Input: part model. Units: mm. Frame: model coordinates. A direction names the side the tool comes from. Coordinates: 2 decimals unless noted, no trailing zeros. Write each loop counter-clockwise with the first axis right and the second up, starting at its lowest first coordinate (ties: lowest second). Pieces come first, ordered by that corner, then holes. Notation, with made-up numbers: M -6,-6 L 32,-6 A15 cw 32,22 Z; hole C 80,28 d8. An arc over 180 degrees is marked long. Write each question's results on one line, items separated by ' | '. Start each with the question number.
1. Section query C-C, the plane x = -120. Output: boundary loops of the cut face in (y, z) (3 decimals).
2. Section query D-D, the plane z = -120. Output: boundary loops of the cut face in (x, y) (3 decimals).
3. First-contact query: pin 1 (6.5 mm diameter, centred on x = 103.92, z = 60, fed in from +Y); pin 2 (3 mm diameter, centred on x = 34, z = -78, fed in from -Y); pin 3 (1.5 mm diameter, centred on y = -21, z = -11.5, fed in from +X). Flat tips, straight axial feed; report the tip coordinate or a pass-through.
4. Ray query, probe 1 along Y at (x, z) = (-45.5, 20); probe 2 along X at (y, z) = (-3, -38); probe 3 along X at (y, z) = (-105.5, -60). Return the intervals inside material, ascending.
5. Pull-direction query (X, two-part tool) for faces 6 (the cylindrical face through (-103.207, -104.918, 65.453)), 7 (the flat face through (38.6, -14.265, -38.699)), 8 (the flat face through (-38.505, -85.33, -38.406)), 9 (the cylindrical face through (-44.74, 4.93, 101.49)); classes: +X half, -X half, draft (parallel to the pull), parting line (faces both ways), or undercut.
6. Set-up query: faces 1 (the flat face through (33.89, -91.01, -40.96)), 2 (the flat face through (38.406, -85.33, -38.505)), 3 (the flat face through (-29, 10, 29)), 4 (the cylindrical face through (98.677, -104.918, -58.348)), 5 (the flat face through (-38.56, -10.79, -31.49)). Return all of +Z, -Z, +X, -X, +Y, -Y with unobstructed straight access to the full face (end or side cutting, diameter ignored); none if empty.
7. Section query A-A, the plane y = 6.5. Count the separate pieces of the cut face and the enclosed holes in it, and give its area (3 significant figures).
8. Section query B-B, the plane z = -74.5. Output: boundary loops of the cut face in (x, y).
```python
from build123d import *

# Parameters (mm, degrees)
SKETCH_1_R                        = 140
SKETCH_1_R_2                      = 30
EXTRUDE_1_DEPTH                   = 10
HOLE_WIZARD_20_0_20_1_AT_2_COUNT  = 2
HOLE_WIZARD_20_0_20_1_AT_2_PITCH  = 127.279220614
HOLE_WIZARD_20_0_20_1_AT_3_COUNT  = 2
HOLE_WIZARD_20_0_20_1_AT_3_PITCH  = 180
HOLE_WIZARD_20_0_20_1_AT_4_COUNT  = 2
HOLE_WIZARD_20_0_20_1_AT_4_PITCH  = 127.279220614
SKETCH_4_R                        = 40
SKETCH_4_R_2                      = 30
EXTRUDE_2_DEPTH                   = 40
EXTRUDE_START                     = -100
SKETCH_6_R                        = 45
SKETCH_6_R_2                      = 30
EXTRUDE_3_DEPTH                   = 100
RIB_6_REACH                       = 223.811
SKETCH_7_WALL_W                   = 483.06475071
SKETCH_7_WALL_H                   = 10
PATTERN_CIRCULAR_1_COUNT          = 4
SKETCH_8_R                        = 131
EXTRUDE_4_DEPTH                   = 10
HOLE_WIZARD_11_0_11_1_D           = 11
HOLE_WIZARD_11_0_11_1_DEPTH       = 10
HOLE_WIZARD_11_0_11_1_CSINK_D     = 11.05
HOLE_WIZARD_11_0_11_1_CSINK_ANGLE = 90
RIB_7_REACH                       = 228.495
SKETCH_11_WALL_W                  = 492.43335657
SKETCH_11_WALL_H                  = 10
PATTERN_CIRCULAR_2_COUNT          = 4


with BuildPart() as part:
    # 草图1 → 凸台-拉伸1 (new body)
    with BuildSketch(Plane(origin=(0, 0, 0), x_dir=(1, 0, 0), z_dir=(0, 1, 0))):
        with Locations(Location((0, 0, 0), (0, 0, 270))):
            Circle(SKETCH_1_R)
        with Locations(Location((0, 0, 0), (0, 0, 270))):
            Circle(SKETCH_1_R_2, mode=Mode.SUBTRACT)
        with BuildLine():
            ThreePointArc((105.655099262, 61), (86.267027305, 86.267027305), (61, 105.655099262))
            ThreePointArc((61, 105.655099262), (44.607695155, 101.262794416), (49, 84.870489571))
            ThreePointArc((49, 84.870489571), (69.296464556, 69.296464556), (84.870489571, 49))
            ThreePointArc((84.870489571, 49), (101.262794416, 44.607695155), (105.655099262, 61))
        make_face(mode=Mode.SUBTRACT)
        with BuildLine():
            ThreePointArc((61, -105.655099262), (86.267027305, -86.267027305), (105.655099262, -61))
            ThreePointArc((105.655099262, -61), (101.262794416, -44.607695155), (84.870489571, -49))
            ThreePointArc((84.870489571, -49), (69.296464556, -69.296464556), (49, -84.870489571))
            ThreePointArc((49, -84.870489571), (44.607695155, -101.262794416), (61, -105.655099262))
        make_face(mode=Mode.SUBTRACT)
        with BuildLine():
            ThreePointArc((-105.655099262, -61), (-86.267027305, -86.267027305), (-61, -105.655099262))
            ThreePointArc((-61, -105.655099262), (-44.607695155, -101.262794416), (-49, -84.870489571))
            ThreePointArc((-49, -84.870489571), (-69.296464556, -69.296464556), (-84.870489571, -49))
            ThreePointArc((-84.870489571, -49), (-101.262794416, -44.607695155), (-105.655099262, -61))
        make_face(mode=Mode.SUBTRACT)
        with BuildLine():
            ThreePointArc((-61, 105.655099262), (-86.267027305, 86.267027305), (-105.655099262, 61))
            ThreePointArc((-105.655099262, 61), (-101.262794416, 44.607695155), (-84.870489571, 49))
            ThreePointArc((-84.870489571, 49), (-69.296464556, 69.296464556), (-49, 84.870489571))
            ThreePointArc((-49, 84.870489571), (-44.607695155, 101.262794416), (-61, 105.655099262))
        make_face(mode=Mode.SUBTRACT)
    extrude(amount=EXTRUDE_1_DEPTH)

    # 草图3 → Ø20.0 (20) 直径孔1 (revolve, cut)
    with BuildSketch(Plane(origin=(0, 10, 90), x_dir=(0, 0, 1), z_dir=(1, 0, 0))):
        Polygon((0, 0), (0, 10), (10, 10), (10, 0.025), (10.025, 0), align=None)
    hole_wizard_20_0_20_1 = revolve(axis=Axis((0, 16.35, 90), (0, -1, 0)), mode=Mode.SUBTRACT)

    # Ø20.0 (20) 直径孔1 at 2: Ø20.0 (20) 直径孔1 ×2
    with Locations(*[Vector(0.7071067811865476, 0, -0.7071067811865476) * (i * HOLE_WIZARD_20_0_20_1_AT_2_PITCH) for i in range(1, HOLE_WIZARD_20_0_20_1_AT_2_COUNT)]):
        add(hole_wizard_20_0_20_1, mode=Mode.SUBTRACT)

    # Ø20.0 (20) 直径孔1 at 3: Ø20.0 (20) 直径孔1 ×2
    with Locations(*[(0, 0, -i * HOLE_WIZARD_20_0_20_1_AT_3_PITCH) for i in range(1, HOLE_WIZARD_20_0_20_1_AT_3_COUNT)]):
        add(hole_wizard_20_0_20_1, mode=Mode.SUBTRACT)

    # Ø20.0 (20) 直径孔1 at 4: Ø20.0 (20) 直径孔1 ×2
    with Locations(*[Vector(-0.7071067811865476, 0, -0.7071067811865476) * (i * HOLE_WIZARD_20_0_20_1_AT_4_PITCH) for i in range(1, HOLE_WIZARD_20_0_20_1_AT_4_COUNT)]):
        add(hole_wizard_20_0_20_1, mode=Mode.SUBTRACT)

    # 草图4 → 凸台-拉伸2 (add)
    with BuildSketch(Plane(origin=(0, 10, 0), x_dir=(1, 0, 0), z_dir=(0, 1, 0))):
        with Locations(Location((0, 0, 0), (0, 0, 270))):
            Circle(SKETCH_4_R)
        with Locations(Location((0, 0, 0), (0, 0, 270))):
            Circle(SKETCH_4_R_2, mode=Mode.SUBTRACT)
    extrude(amount=EXTRUDE_2_DEPTH)

    # 草图6 → 凸台-拉伸3 (add)
    with BuildSketch(Plane(origin=(0, 0, 0), x_dir=(1, 0, 0), z_dir=(0, 1, 0)).offset(EXTRUDE_START)):
        with Locations(Location((0, 0, 0), (0, 0, 270))):
            Circle(SKETCH_6_R)
        with Locations(Location((0, 0, 0), (0, 0, 270))):
            Circle(SKETCH_6_R_2, mode=Mode.SUBTRACT)
    extrude(amount=EXTRUDE_3_DEPTH)

    # 草图7 wall → 筋6 (add, up to next)
    with BuildSketch(Plane(origin=(38.537319575, -14.5, 38.537319575), x_dir=(-0.396579526667, -0.827918690487, -0.396579526667), z_dir=(0.585426920314, -0.560848145172, 0.585426920314)), mode=Mode.PRIVATE) as rib_6_sk1:
        Rectangle(SKETCH_7_WALL_W, SKETCH_7_WALL_H)
    rib_6_tool1 = extrude(rib_6_sk1.sketch, amount=-RIB_6_REACH, mode=Mode.PRIVATE) - part.part
    rib_6 = rib_6_tool1.solids().sort_by_distance((38.537319575, -14.5, 38.537319575))[0]
    add(rib_6)

    # 阵列(圆周)1: 筋6 ×4 about axis
    pattern_circular_1_axis = Axis((0, 0, 0), (0, 1, 0))
    for i in range(1, PATTERN_CIRCULAR_1_COUNT):
        add(rib_6.rotate(pattern_circular_1_axis, i * 360 / PATTERN_CIRCULAR_1_COUNT))

    # 草图8 → 凸台-拉伸4 (add)
    with BuildSketch(Plane.XZ.offset(100)):
        with Locations(Location((0, 0, 0), (0, 0, 270))):
            Circle(SKETCH_8_R)
        with BuildLine():
            ThreePointArc((32.491913616, 89.270798975), (0, 95), (-32.491913616, 89.270798975))
            ThreePointArc((-32.491913616, 89.270798975), (-41.457000778, 70.045107513), (-22.231309316, 61.080020351))
            ThreePointArc((-22.231309316, 61.080020351), (0, 65), (22.231309316, 61.080020351))
            ThreePointArc((22.231309316, 61.080020351), (41.457000778, 70.045107513), (32.491913616, 89.270798975))
        make_face(mode=Mode.SUBTRACT)
        with BuildLine():
            ThreePointArc((89.270798975, -32.491913616), (95, 0), (89.270798975, 32.491913616))
            ThreePointArc((89.270798975, 32.491913616), (70.045107513, 41.457000778), (61.080020351, 22.231309316))
            ThreePointArc((61.080020351, 22.231309316), (65, 0), (61.080020351, -22.231309316))
            ThreePointArc((61.080020351, -22.231309316), (70.045107513, -41.457000778), (89.270798975, -32.491913616))
        make_face(mode=Mode.SUBTRACT)
        with BuildLine():
            ThreePointArc((-32.491913616, -89.270798975), (0, -95), (32.491913616, -89.270798975))
            ThreePointArc((32.491913616, -89.270798975), (41.457000778, -70.045107513), (22.231309316, -61.080020351))
            ThreePointArc((22.231309316, -61.080020351), (0, -65), (-22.231309316, -61.080020351))
            ThreePointArc((-22.231309316, -61.080020351), (-41.457000778, -70.045107513), (-32.491913616, -89.270798975))
        make_face(mode=Mode.SUBTRACT)
        with BuildLine():
            ThreePointArc((-89.270798975, 32.491913616), (-95, 0), (-89.270798975, -32.491913616))
            ThreePointArc((-89.270798975, -32.491913616), (-70.045107513, -41.457000778), (-61.080020351, -22.231309316))
            ThreePointArc((-61.080020351, -22.231309316), (-65, 0), (-61.080020351, 22.231309316))
            ThreePointArc((-61.080020351, 22.231309316), (-70.045107513, 41.457000778), (-89.270798975, 32.491913616))
        make_face(mode=Mode.SUBTRACT)
    extrude(amount=EXTRUDE_4_DEPTH)

    # Ø11.0 (11) 直径孔1
    with Locations(Plane.XZ.offset(110)):
        with Locations((0, 0), (0, 120), (60, 103.923048454), (103.923048454, 60), (120, 0), (103.923048454, -60), (60, -103.923048454), (0, -120), (-60, -103.923048454), (-103.923048454, -60), (-120, 0), (-103.923048454, 60), (-60, 103.923048454)):
            CounterSinkHole(HOLE_WIZARD_11_0_11_1_D / 2, HOLE_WIZARD_11_0_11_1_CSINK_D / 2, depth=HOLE_WIZARD_11_0_11_1_DEPTH, counter_sink_angle=HOLE_WIZARD_11_0_11_1_CSINK_ANGLE)

    # 草图11 wall → 筋7 (add, up to next)
    with BuildSketch(Plane(origin=(38.537319575, -85.5, 38.537319575), x_dir=(0.396579526667, -0.827918690487, 0.396579526667), z_dir=(0.585426920314, 0.560848145172, 0.585426920314)), mode=Mode.PRIVATE) as rib_7_sk1:
        Rectangle(SKETCH_11_WALL_W, SKETCH_11_WALL_H)
    rib_7_tool1 = extrude(rib_7_sk1.sketch, amount=-RIB_7_REACH, mode=Mode.PRIVATE) - part.part
    rib_7 = rib_7_tool1.solids().sort_by_distance((38.537319575, -85.5, 38.537319575))[0]
    add(rib_7)

    # 阵列(圆周)2: 筋7 ×4 about axis
    pattern_circular_2_axis = Axis((0, 0, 0), (0, 1, 0))
    for i in range(1, PATTERN_CIRCULAR_2_COUNT):
        add(rib_7.rotate(pattern_circular_2_axis, i * 360 / PATTERN_CIRCULAR_2_COUNT))


solid = part.part
```
Answer:
1) outline: M -110,-52.545 L -100,-52.545 L -100,-5.5 L -109.975,-5.5 L -110,-5.525 Z; M -110,5.525 L -109.975,5.5 L -100,5.5 L -100,52.545 L -110,52.545 Z; M 0,-72.111 L 10,-72.111 L 10,72.111 L 0,72.111 Z
2) outline: M -72.111,0 L 72.111,0 L 72.111,10 L -72.111,10 Z; M -52.545,-110 L -5.525,-110 L -5.5,-109.975 L -5.5,-100 L -52.545,-100 Z; M 5.5,-109.975 L 5.525,-110 L 52.545,-110 L 52.545,-100 L 5.5,-100 Z
3) pin 1: y = 10 | pin 2: y = 0 | pin 3: x = 43.7
4) probe 1: -110 to -100, 0 to 10 | probe 2: -45.07 to -30.93, -24.1 to 24.1, 30.93 to 45.07 | probe 3: -116.45 to -109.42, -98.42 to 98.42, 109.42 to 116.45
5) face 6: undercut | face 7: +X half | face 8: -X half | face 9: undercut
6) face 1: -Z | face 2: -Z, +X | face 3: +Y | face 4: -Y | face 5: -X
7) separate pieces: 1 | enclosed holes: 9 | area: 50,200 mm^2
8) outline: M -118.53,0 L -96.61,0 L -96.61,10 L -118.53,10 Z; M -107.75,-110 L -42.35,-110 L -42.35,-100 L -107.75,-100 Z; M -63.67,0 L 63.67,0 L 63.67,10 L -63.67,10 Z; M 42.35,-110 L 107.75,-110 L 107.75,-100 L 42.35,-100 Z; M 96.61,0 L 118.53,0 L 118.53,10 L 96.61,10 Z
